Answer from the drawing. Dimensions are ordinates in mm from the lowest x, y and z of the part. Coordinates: 2 decimals unless noted, no trailing zeros. Write each loop counter-clockwise with the first axis right and the second up, starting at its lowest first coordinate (ties: lowest second). Pieces come first, ordered by that corner, then holes. Notation, with made-up numbers: (9, 3) -> (40, 3) arc R30 cw to (40, 28) -> close; hole circle Ø9 at (73, -21). An arc over 180 degrees is marked (long way). Use CSV: the item, a comma, the result in double quotes.
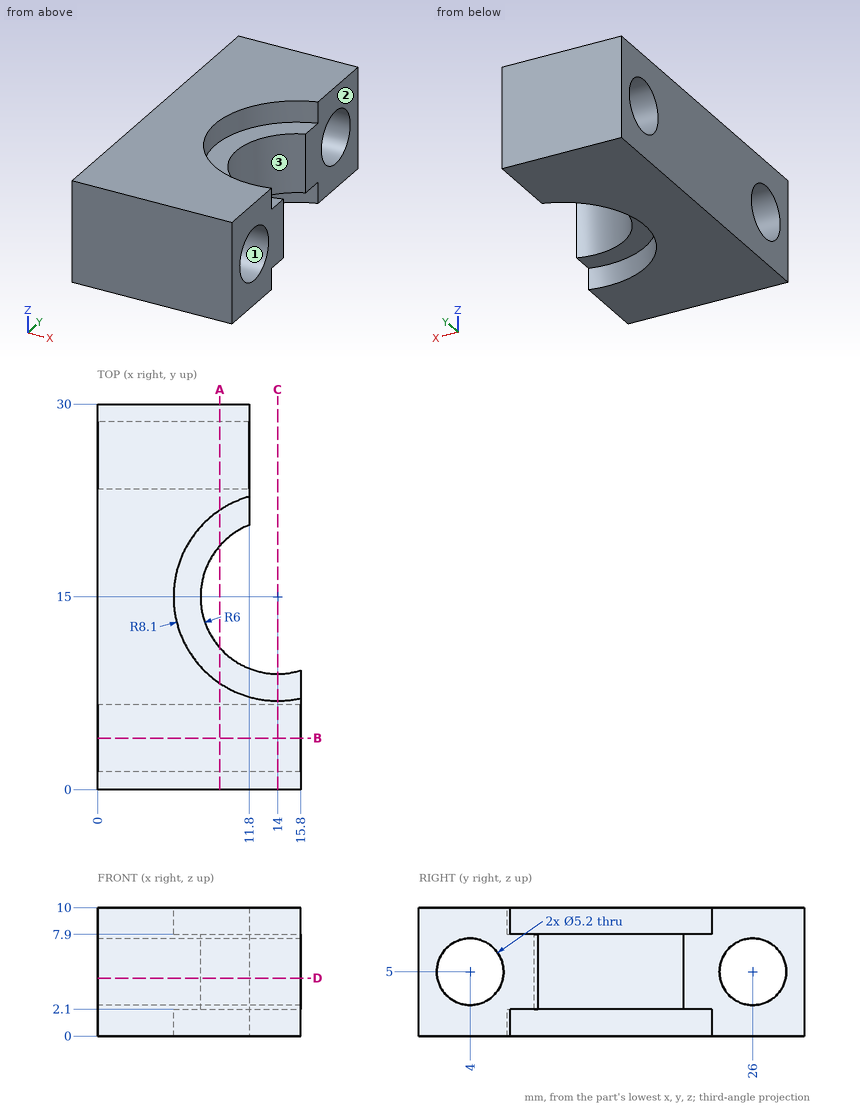
1. Each of these flat-tipped pins is pushed along its axis until it touches: pin 1 Ø5 at (x, y) = (10.5, 18.5) entering from -Z; pin 2 Ø4 at (y, z) = (4, 5) entering from -X; pin 3 Ø3 at (y, z) = (26.5, 7) entering from +X; pin 4 Ø5 at (x, y) = (9, 15.5) entering from +Z. Where does it stop, or does it pass through?
Solutions:
pin 1,"stops at z = 2.1"
pin 2,"passes through"
pin 3,"stops at x = 11.8"
pin 4,"stops at z = 7.9"
2. Find the intervals of material crossed by line 1 along Y through (x, z) = (8.5, 5.5); line 2 along Y through (x, z) = (2.5, 7); line 3 along Z through (x, y) = (3, 26), in increasing order.
Solutions:
line 1,"y = 0 to 1.45, 6.55 to 12.6, 17.4 to 23.45, 28.55 to 30"
line 2,"y = 0 to 2.34, 5.66 to 24.34, 27.66 to 30"
line 3,"z = 0 to 2.4, 7.6 to 10"
3. A cutting plane is placed at A-A (x = 9.5). Give the vertices of the cut face in (y, z), and give its area (3 significant figures).
Solutions:
outline,"(0, 0) -> (8.27, 0) -> (8.27, 2.1) -> (11.03, 2.1) -> (11.03, 7.9) -> (8.27, 7.9) -> (8.27, 10) -> (0, 10) -> close; (18.97, 2.1) -> (21.73, 2.1) -> (21.73, 0) -> (30, 0) -> (30, 10) -> (21.73, 10) -> (21.73, 7.9) -> (18.97, 7.9) -> close; hole circle Ø5.2 at (4, 5); hole circle Ø5.2 at (26, 5)"
area,"155 mm^2"
4. A cutting plane is placed at C-C (x = 14). Give the vertices of the cut face in (y, z), and give its area (3 significant figures).
Solutions:
outline,"(0, 0) -> (6.9, 0) -> (6.9, 2.1) -> (9, 2.1) -> (9, 7.9) -> (6.9, 7.9) -> (6.9, 10) -> (0, 10) -> close; hole circle Ø5.2 at (4, 5)"
area,"59.9 mm^2"
5. For a pull along X with two mould halves and no side action, classify the marked faces 1, 2 and 3 as pulls with the +X half, pulls with the -X half, needs draft (parallel to the pull), parting line crosses it, or undercut.
Solutions:
face 1,"needs draft"
face 2,"pulls with the +X half"
face 3,"undercut"
6. A cutting plane is placed at D-D (z = 4.5). Give the vertices of the cut face in (x, y), and give its area (3 significant figures).
Solutions:
outline,"(0, 0) -> (15.8, 0) -> (15.8, 1.45) -> (0, 1.45) -> close; (0, 6.55) -> (15.8, 6.55) -> (15.8, 9.28) arc R6 cw to (11.8, 20.58) -> (11.8, 23.45) -> (0, 23.45) -> close; (0, 28.55) -> (11.8, 28.55) -> (11.8, 30) -> (0, 30) -> close"
area,"219 mm^2"
7. A cutting plane is placed at B-B (y = 4). Give the vertices of the cut face in (x, z), and give its area (3 significant figures).
Solutions:
outline,"(0, 0) -> (15.8, 0) -> (15.8, 2.4) -> (0, 2.4) -> close; (0, 7.6) -> (15.8, 7.6) -> (15.8, 10) -> (0, 10) -> close"
area,"75.8 mm^2"
